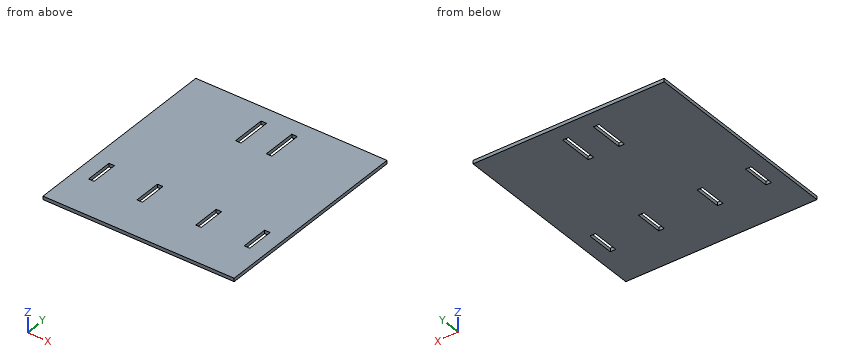
```python
from build123d import *

# Parameters (mm, degrees)
SKETCH1_W           = 280
SKETCH1_H           = 300
BOSS_EXTRUDE1_DEPTH = 5
SKETCH2_W           = 8
SKETCH2_H           = 40
SKETCH2_H_2         = 50
CUT_EXTRUDE1_DEPTH  = 332.096662623


with BuildPart() as part:
    # Sketch1 → Boss-Extrude1 (new body)
    with BuildSketch(Plane.XY):
        with Locations((0, 150)):
            Rectangle(SKETCH1_W, SKETCH1_H)
    extrude(amount=BOSS_EXTRUDE1_DEPTH)

    # Sketch2 → Cut-Extrude1 (cut, through all)
    with BuildSketch(Plane(origin=(0, 0, 0), x_dir=(-1, 0, 0), z_dir=(0, 0, -1))):
        with Locations((-114, 80)):
            Rectangle(SKETCH2_W, SKETCH2_H)
        with Locations((-43, 80)):
            Rectangle(SKETCH2_W, SKETCH2_H)
        with Locations((43, 80)):
            Rectangle(SKETCH2_W, SKETCH2_H)
        with Locations((114, 80)):
            Rectangle(SKETCH2_W, SKETCH2_H)
        with Locations((-22.5, 251)):
            Rectangle(SKETCH2_W, SKETCH2_H_2)
        with Locations((22.5, 251)):
            Rectangle(SKETCH2_W, SKETCH2_H_2)
    extrude(amount=-CUT_EXTRUDE1_DEPTH, mode=Mode.SUBTRACT)


solid = part.part
```
For this review, take the finished solid that the model builds, in its own axes (mm). Coordinates: 2 decimals unless noted, no trailing zeros. Order: outer loops, then holes, each group sorted by start corner. A loop starts at its lowest first (then second) coordinate and runs counter-clockwise, first axis right, second up. Notation, with made-up numbers: (60, 19) - (114, 19) arc R27 ccw to (114, 57) - close; hole circle Ø7 at (57, -5). An arc over 180 degrees is marked (long way). Answer as a JSON object with one key per item and string values. Group by question number.
1. We need section A-A on y = 266. State the section outline as (x, z) points.
2. Clearance check with a flat-ended pin moving along its axis: P1, Ø12, axis at x = -52, y = 155.5, coming from the -Z side. State where the tip first meets the part, or that it passes through.
3. For probe 1 along X at (y, z) = (267.5, 1.8); probe 2 along Y at (x, z) = (117.5, 3), list the stretches that pass through material, from the lowest coordinate up.
4. We need section B-B on z = 4. State the section outline as (x, y) points, then the cut area to 3 significant figures.
Final values:
{
 "1": {"outline": "(-140, 0) - (-26.5, 0) - (-26.5, 5) - (-140, 5) - close; (-18.5, 0) - (18.5, 0) - (18.5, 5) - (-18.5, 5) - close; (26.5, 0) - (140, 0) - (140, 5) - (26.5, 5) - close"},
 "2": {"P1": "z = 0"},
 "3": {"probe 1": "-140 to -26.5, -18.5 to 18.5, 26.5 to 140", "probe 2": "0 to 60, 100 to 300"},
 "4": {"outline": "(-140, 0) - (140, 0) - (140, 300) - (-140, 300) - close; hole (-118, 60) - (-110, 60) - (-110, 100) - (-118, 100) - close; hole (-47, 60) - (-39, 60) - (-39, 100) - (-47, 100) - close; hole (-26.5, 226) - (-18.5, 226) - (-18.5, 276) - (-26.5, 276) - close; hole (18.5, 226) - (26.5, 226) - (26.5, 276) - (18.5, 276) - close; hole (39, 60) - (47, 60) - (47, 100) - (39, 100) - close; hole (110, 60) - (118, 60) - (118, 100) - (110, 100) - close", "area": "81,900 mm²"}
}
